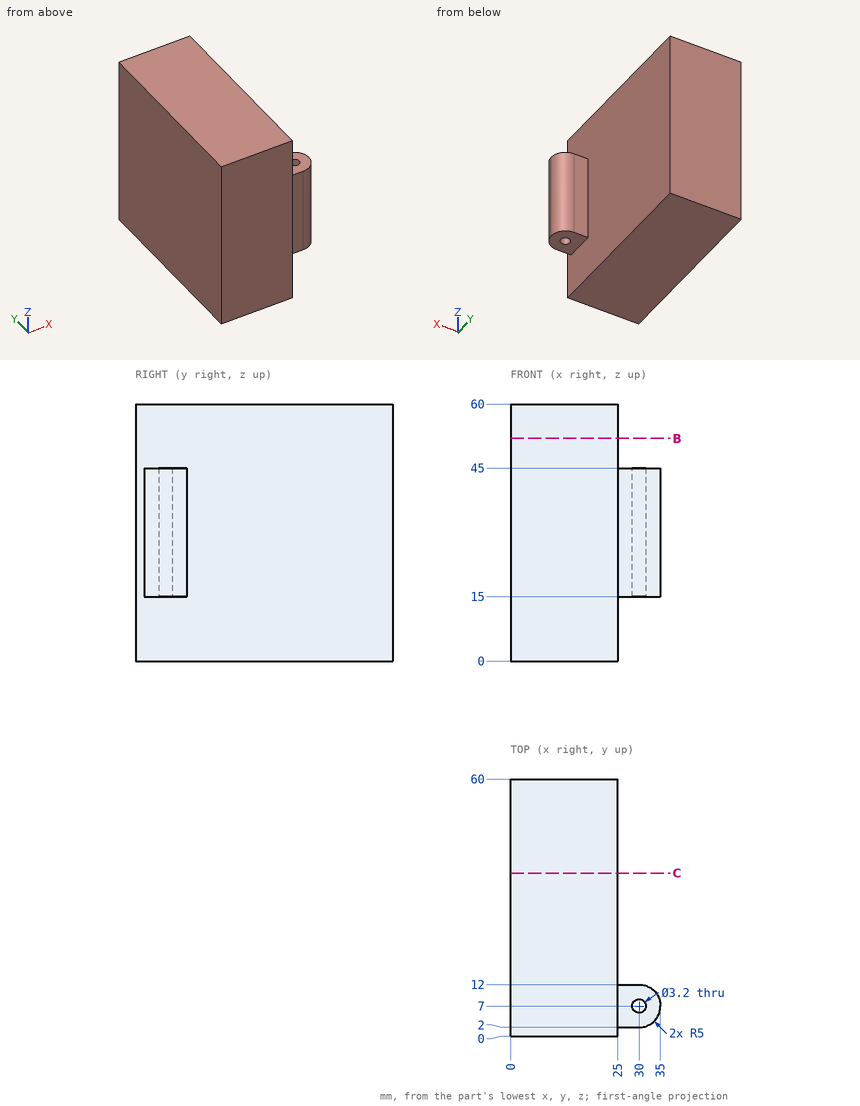
Study the drawing (mm; zero at the part's minimum x, y, z) and answer. Give positions to 0.01 mm unless a question says otherwise; leave off trailing zeros. Write each loop counter-clockwise with the first axis right and the second up, starting at its lowest first coordinate (ties: lowest second). Pieces come first, ordered by that corner, then holes. Notation, with made-up numbers: (63.25, -4) -> (120.25, -4) arc R23 ccw to (120.25, 24) -> close; hole circle Ø8 at (71.25, 87). An arc over 180 degrees is marked (long way). Answer in a Markdown table with one row per item.
1) Section B-B on z = 52 is taken. Give the vertices of the cut face in (x, y).
Results list:
| item | result |
|---|---|
| outline | (0, 0) -> (25, 0) -> (25, 60) -> (0, 60) -> close |
2) Straight lines are drawn through the part: line 1 (Y direction, x = 30, z = 31.25); line 2 (X direction, y = 24, z = 32.5); line 3 (Z direction, x = 28, y = 6). For each, find the intervals that lie inside material, in ascending order. Write a range as [from, to].
Results list:
| item | result |
|---|---|
| line 1 | [2, 5.4], [8.6, 12] |
| line 2 | [0, 25] |
| line 3 | [15, 45] |
3) Each of these flat-tipped pins is pushed along its axis until it touches: pin 1 Ø2.5 at (x, z) = (27.5, 37) entering from -Y; pin 2 Ø10 at (y, z) = (27.5, 44.5) entering from +X; pin 3 Ø4 at (x, z) = (27.5, 24.5) entering from +Y. Where does it stop, or does it pass through?
Results list:
| item | result |
|---|---|
| pin 1 | y = 2 |
| pin 2 | x = 25 |
| pin 3 | y = 12 |
